Verification items for the finished model (mm, model axes). A direction names the side the tool comes from. Round coordinates to 2 decimals unless told otherwise and drop trailing zeros. Loops run counter-clockwise (first coordinate to the right, second up) from the corner with the lowest first, then second, coordinate; pieces in that order, holes last. Notation, with made-up numbers: M 59.25,-34 L 66.25,-34 A16 cw 66.25,-18 Z; hole C 78.5,-11 d8. An arc over 180 degrees is marked long. One line per item, written item: value.
from build123d import *

# Parameters (mm, degrees)
F2_R = 9.5


with BuildPart() as f3:
    # F3: sweep along a path in F0
    with BuildLine(Plane.XZ) as f3_path:
        Line((-60.6934127808, 0), (-60.6934127808, 720.5))
        ThreePointArc((-60.6934127808, 720.5), (-46.0487518401, 755.8553390593), (-10.6934127808, 770.5))
        Line((-10.6934127808, 770.5), (220.3065872192, 770.5))
        ThreePointArc((220.3065872192, 770.5), (255.6619262786, 755.8553390593), (270.3065872192, 720.5))
        Line((270.3065872192, 720.5), (270.3065872192, 0))
    # F2 (on face) → F3 (sweep)
    with BuildSketch(Plane.XY):
        with Locations((-60.6934127808, 0)):
            Circle(F2_R)
    sweep(path=f3_path.line)


solid = f3.part
(1) Depth check by flat-ended pin: pin 1 Ø1.5 at (y, z) = (-3.5, 338) entering from -X; pin 2 Ø1.5 at (x, y) = (117.5, -2.5) entering from -Z; pin 3 Ø1 at (y, z) = (-6.5, 175) entering from +X. Enter the tip coordinate at first touch or a pass-through.
Completed:
pin 1: stops at x = -69.79
pin 2: stops at z = 761.16
pin 3: stops at x = 277.67
(2) Sectioned sample at B-B on z = 538.5. Enter the section's corners in (x, y).
Completed:
outline: C -60.69,0 d19; C 270.31,0 d19
(3) Mould release check, pull along X, two halves, no side actions. Record for faces 4 (the face through (-68.232, -5.781, 365.294)), 5 (the face through (-61, 0, 0)): +X half, -X half, draft (parallel to the pull), parting line (faces both ways), or undercut.
Completed:
face 4: undercut
face 5: draft
(4) Sectioned sample at C-C on x = 141. Enter the section's corners in (y, z).
Completed:
outline: C 0,770.5 d19
(5) Sectioned sample at A-A on y = 0. Enter the section's corners in (x, z), and give its area (3 significant figures).
Completed:
outline: M -70.19,0 L -51.19,0 L -51.19,720.5 A40.5 cw -10.69,761 L 220.31,761 A40.5 cw 260.81,720.5 L 260.81,0 L 279.81,0 L 279.81,720.5 A59.5 ccw 220.31,780 L -10.69,780 A59.5 ccw -70.19,720.5 Z
area: 34,800 mm^2
(6) Thickness scan on L1, parallel to X at y = 1.25, z = 477; L2, parallel to Z at x = 96.5, y = 1.25; L3, parallel to X at y = 4.5, z = 636.5. Record the ranges inside material, lowest first. Write a range as from..to.
Completed:
L1: x = -70.11..-51.28, 260.89..279.72
L2: z = 761.08..779.92
L3: x = -69.06..-52.33, 261.94..278.67
(7) Tool access check on faces 1 (the face through (261.53, -3.64, 355.21)), 2 (the face through (270, 0, 0)), 3 (the face through (106, 0, 780)). Record the directions out of +Z, -Z, +X, -X, +Y, -Y that give a thin tool (end or side, any length) a straight path to the whole face; none if there is none.
Completed:
face 1: -Z
face 2: -Z, +X, -X, +Y, -Y
face 3: none
